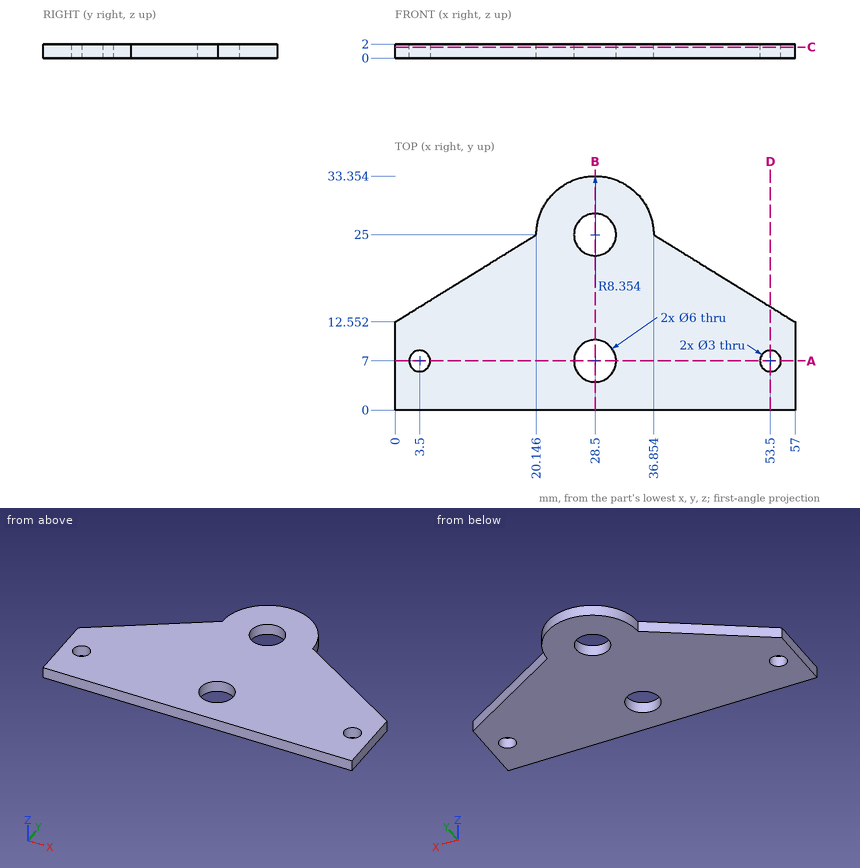
Job drawing, mm, ordinate dimensions from the low corner. One solid piece. Round coordinates to 2 decimals unless told otherwise and drop trailing zeros. Loops run counter-clockwise (first coordinate to the right, second up) from the corner with the lowest first, then second, coordinate; pieces in that order, holes last.
(1) Cut at C-C (z = 1.55). Give the cut face in (x, y).
(2) Cut at D-D (x = 53.5). Give the cut face in (y, z) (1 decimal).
(3) Wall check: line 1 along Y through (x, z) = (28.5, 0.6); line 2 along X through (y, z) = (6, 1.4); line 3 along Y through (x, z) = (3.5, 1.4) (1 decimal). Give the ranges that are in metal, low to high.
(4) Cut at A-A (y = 7). Give the cut face in (x, z).
(5) Cut at B-B (x = 28.5). Give the cut face in (y, z), plus the area to 3 significant figures.
Findings below:
1. outline: (0, 0) - (57, 0) - (57, 12.55) - (36.85, 25) arc R8.35 ccw to (20.15, 25) - (0, 12.55) - close; hole circle Ø3 at (3.5, 7); hole circle Ø6 at (28.5, 7); hole circle Ø6 at (28.5, 25); hole circle Ø3 at (53.5, 7)
2. outline: (0, 0) - (5.5, 0) - (5.5, 2) - (0, 2) - close; (8.5, 0) - (14.7, 0) - (14.7, 2) - (8.5, 2) - close
3. line 1: y = 0 to 4, 10 to 22, 28 to 33.35
3. line 2: x = 0 to 2.38, 4.62 to 25.67, 31.33 to 52.38, 54.62 to 57
3. line 3: y = 0 to 5.5, 8.5 to 14.7
4. outline: (0, 0) - (2, 0) - (2, 2) - (0, 2) - close; (5, 0) - (25.5, 0) - (25.5, 2) - (5, 2) - close; (31.5, 0) - (52, 0) - (52, 2) - (31.5, 2) - close; (55, 0) - (57, 0) - (57, 2) - (55, 2) - close
5. outline: (0, 0) - (4, 0) - (4, 2) - (0, 2) - close; (10, 0) - (22, 0) - (22, 2) - (10, 2) - close; (28, 0) - (33.35, 0) - (33.35, 2) - (28, 2) - close
5. area: 42.7 mm2
